Geometry check sheet. Reference: the model listing, model coordinates, mm. A direction names the side the tool comes from. Give positions to 0.01 mm unless a question says otherwise; leave off trailing zeros. Write each loop counter-clockwise with the first axis right and the second up, starting at its lowest first coordinate (ties: lowest second). Pieces come first, ordered by that corner, then holes. Notation, with made-up numbers: (-20.75, -38.75) - (4.25, -38.75) arc R28 cw to (4.25, -1.75) - close; hole circle Ø1 at (16, 1.25). An arc over 180 degrees is marked (long way). Use a Markdown table: item, result.
```python
from build123d import *

# Parameters (mm, degrees)
F0_W     = 38.5
F0_H     = 22.8
F1_DEPTH = 12.55
F2_R     = 2
F3_T     = -0.5


with BuildPart() as f1:
    # F0 (on Front) → F1 (new body)
    with BuildSketch(Plane.XZ):
        with Locations((-26.358417, 20.3031)):
            Rectangle(F0_W, F0_H)
    extrude(amount=F1_DEPTH)

    # F2
    f2_edges = [f1.edges().sort_by_distance(p)[0] for p in [
        (-45.608417, -12.55, 20.3031),
        (-45.608417, 0, 20.3031),
        (-7.108417, -12.55, 20.3031),
        (-7.108417, 0, 20.3031),
        (-26.358417, -12.55, 31.7031),
        (-7.108417, -6.275, 31.7031),
        (-26.358417, 0, 31.7031),
        (-45.608417, -6.275, 31.7031),
    ]]
    fillet(f2_edges, radius=F2_R)

    # F3
    f3_openings = [f1.faces().sort_by_distance(p)[0] for p in [
        (-26.358417, -6.275, 8.9031),
    ]]
    offset(amount=F3_T, openings=f3_openings)


solid = f1.part
```
1) Section check C-C on y = -6. Record the boundary of the cut face in (x, z), then the cut area to 3 significant figures.
Working result:
| item | result |
|---|---|
| outline | (-45.61, 8.9) - (-45.11, 8.9) - (-45.11, 29.7) arc R1.5 cw to (-43.61, 31.2) - (-9.11, 31.2) arc R1.5 cw to (-7.61, 29.7) - (-7.61, 8.9) - (-7.11, 8.9) - (-7.11, 29.7) arc R2 ccw to (-9.11, 31.7) - (-43.61, 31.7) arc R2 ccw to (-45.61, 29.7) - close |
| area | 40.8 mm² |
2) Material ranges on L1, parallel to Y at x = -13, z = 11.25; L2, parallel to X at y = -9.5, z = 19.25; L3, parallel to Z at x = -33, y = -9.25, recorded low to high. Write a range as from..to.
Working result:
| item | result |
|---|---|
| L1 | y = -12.55..-12.05, -0.5..0 |
| L2 | x = -45.61..-45.11, -7.61..-7.11 |
| L3 | z = 31.2..31.7 |
3) Section check B-B on x = -26.5. Record the boundary of the cut face in (y, z).
Working result:
| item | result |
|---|---|
| outline | (-12.55, 8.9) - (-12.05, 8.9) - (-12.05, 29.7) arc R1.5 cw to (-10.55, 31.2) - (-2, 31.2) arc R1.5 cw to (-0.5, 29.7) - (-0.5, 8.9) - (0, 8.9) - (0, 29.7) arc R2 ccw to (-2, 31.7) - (-10.55, 31.7) arc R2 ccw to (-12.55, 29.7) - close |
4) Depth check by flat-ended pin: P1, Ø4.5, axis at x = -25.5, y = -5.5, coming from the -Z side. Enter the tip coordinate at first touch or a pass-through.
Working result:
| item | result |
|---|---|
| P1 | stops at z = 31.2 |
5) Set-up check for faces 1 (the flat face through (-27, -0.5, 19)), 2 (the cylindrical face through (-45.038, -11.949, 19.449)): record each of +Z, -Z, +X, -X, +Y, -Y from which the full face is reachable in a straight line by a thin tool's end or side.
Working result:
| item | result |
|---|---|
| face 1 | -Z |
| face 2 | +Z, -Z, -X, -Y |
6) Mould release check, pull along X, two halves, no side actions. Record for faces 3 (the flat face through (-7.108, -6, 19)), 4 (the cylindrical face through (-45.04, -6.33, 31.1)), 5 (the flat face through (-7.608, -6, 19)), 6 (the flat face through (-27, -12.55, 19)): pulls with the +X half, pulls with the -X half, needs draft (parallel to the pull), parting line crosses it, or undercut.
Working result:
| item | result |
|---|---|
| face 3 | pulls with the +X half |
| face 4 | pulls with the -X half |
| face 5 | undercut |
| face 6 | needs draft |
7) Section check A-A on z = 28.5. Record the boundary of the cut face in (x, y).
Working result:
| item | result |
|---|---|
| outline | (-45.61, -10.55) arc R2 ccw to (-43.61, -12.55) - (-9.11, -12.55) arc R2 ccw to (-7.11, -10.55) - (-7.11, -2) arc R2 ccw to (-9.11, 0) - (-43.61, 0) arc R2 ccw to (-45.61, -2) - close; hole (-45.11, -10.55) arc R1.5 ccw to (-43.61, -12.05) - (-9.11, -12.05) arc R1.5 ccw to (-7.61, -10.55) - (-7.61, -2) arc R1.5 ccw to (-9.11, -0.5) - (-43.61, -0.5) arc R1.5 ccw to (-45.11, -2) - close |
